The model under review builds one solid part; all positions refer to its coordinate system, in mm. Face numbers are marked on the shaded views. A direction names the side the tool comes from. Give positions to 0.01 mm unless a question says otherwise; leave off trailing zeros. Order: outer loops, then holes, each group sorted by start corner. A loop starts at its lowest first (then second) coordinate and runs counter-clockwise, first axis right, second up. Notation, with made-up numbers: (-23.75, 83) - (6.25, 83) arc R12 ccw to (6.25, 99) - close; hole circle Ø4 at (46, 24). An arc over 180 degrees is marked (long way). Answer as CSV lines item,"result". Start each with the question number.
from build123d import *

# Parameters (mm, degrees)
SKETCH1_R           = 9.5
BOSS_EXTRUDE1_DEPTH = 68
SKETCH2_R           = 8
BOSS_EXTRUDE2_DEPTH = 28
SKETCH3_R           = 7
BOSS_EXTRUDE3_DEPTH = 22
SKETCH4_R           = 6
BOSS_EXTRUDE4_DEPTH = 10
SKETCH5_R           = 37.5
BOSS_EXTRUDE5_DEPTH = 1.5
SKETCH6_R           = 12.5
SKETCH6_R_2         = 7
BOSS_EXTRUDE6_DEPTH = 17.5
FILLET1_R           = 6
BOSS_EXTRUDE7_DEPTH = 14
FILLET2_R           = 3


with BuildPart() as part:
    # Sketch1 → Boss-Extrude1 (new body)
    with BuildSketch(Plane.XY):
        Circle(SKETCH1_R)
    extrude(amount=BOSS_EXTRUDE1_DEPTH)

    # Sketch2 → Boss-Extrude2 (add)
    with BuildSketch(Plane.XY.offset(68)):
        Circle(SKETCH2_R)
    extrude(amount=BOSS_EXTRUDE2_DEPTH)

    # Sketch3 → Boss-Extrude3 (add)
    with BuildSketch(Plane.XY.offset(96)):
        Circle(SKETCH3_R)
    extrude(amount=BOSS_EXTRUDE3_DEPTH)

    # Sketch4 → Boss-Extrude4 (add)
    with BuildSketch(Plane.XY.offset(118)):
        Circle(SKETCH4_R)
    extrude(amount=BOSS_EXTRUDE4_DEPTH)

    # Sketch5 → Boss-Extrude5 (add)
    with BuildSketch(Plane(origin=(0, 0, 0), x_dir=(-1, 0, 0), z_dir=(0, 0, -1))):
        Circle(SKETCH5_R)
    extrude(amount=BOSS_EXTRUDE5_DEPTH)

    # Sketch6 → Boss-Extrude6 (add)
    with BuildSketch(Plane(origin=(0, 0, -1.5), x_dir=(-1, 0, 0), z_dir=(0, 0, -1))):
        Circle(SKETCH6_R)
        Circle(SKETCH6_R_2, mode=Mode.SUBTRACT)
    extrude(amount=BOSS_EXTRUDE6_DEPTH)

    # Fillet1
    fillet1_edges = [part.edges().sort_by_distance(p)[0] for p in [
        (12.5, 0, -1.5),
    ]]
    fillet(fillet1_edges, radius=FILLET1_R)

    # Sketch8 → Boss-Extrude7 (add)
    with BuildSketch(Plane.XY):
        with BuildLine():
            ThreePointArc((-14.519262929, -12.255243939), (-13.410586975, -13.459426325), (-12.202382266, -14.563717487))
            ThreePointArc((-12.202382266, -14.563717487), (-23.134563913, -16.979972169), (-34.212072677, -15.355262394))
            ThreePointArc((-34.212072677, -15.355262394), (-34.993730727, -13.479199154), (-35.672601083, -11.563543228))
            ThreePointArc((-35.672601083, -11.563543228), (-25.163804407, -13.985042516), (-14.519262929, -12.255243939))
        make_face()
        with BuildLine():
            ThreePointArc((7.821978348, 36.675150371), (0.470500112, 28.78501513), (-3.353721116, 18.70167251))
            ThreePointArc((-3.353721116, 18.70167251), (-4.95091163, 18.343622162), (-6.511358184, 17.849431772))
            ThreePointArc((-6.511358184, 17.849431772), (-3.137805297, 28.525106139), (3.807989024, 37.306155251))
            ThreePointArc((3.807989024, 37.306155251), (5.823536473, 37.045059359), (7.821978348, 36.675150371))
        make_face()
        with BuildLine():
            ThreePointArc((-27.850622735, 25.111607143), (-24.693304295, 14.799972614), (-17.872984045, 6.446428571))
            ThreePointArc((-17.872984045, 6.446428571), (-18.361498605, 4.884195838), (-18.71374045, 3.285714286))
            ThreePointArc((-18.71374045, 3.285714286), (-26.27236921, 11.54513397), (-30.404083653, 21.950892857))
            ThreePointArc((-30.404083653, 21.950892857), (-29.170194253, 23.565860206), (-27.850622735, 25.111607143))
        make_face()
        with BuildLine():
            ThreePointArc((35.672601083, 11.563543228), (25.163804407, 13.985042516), (14.519262929, 12.255243939))
            ThreePointArc((14.519262929, 12.255243939), (13.410586975, 13.459426325), (12.202382266, 14.563717487))
            ThreePointArc((12.202382266, 14.563717487), (23.134563913, 16.979972169), (34.212072677, 15.355262394))
            ThreePointArc((34.212072677, 15.355262394), (34.993730727, 13.479199154), (35.672601083, 11.563543228))
        make_face()
        with BuildLine():
            ThreePointArc((27.850622735, -25.111607143), (24.693304295, -14.799972614), (17.872984045, -6.446428571))
            ThreePointArc((17.872984045, -6.446428571), (18.361498605, -4.884195838), (18.71374045, -3.285714286))
            ThreePointArc((18.71374045, -3.285714286), (26.27236921, -11.54513397), (30.404083653, -21.950892857))
            ThreePointArc((30.404083653, -21.950892857), (29.170194253, -23.565860206), (27.850622735, -25.111607143))
        make_face()
        with BuildLine():
            ThreePointArc((-7.821978348, -36.675150371), (-0.470500112, -28.78501513), (3.353721116, -18.70167251))
            ThreePointArc((3.353721116, -18.70167251), (4.95091163, -18.343622162), (6.511358184, -17.849431772))
            ThreePointArc((6.511358184, -17.849431772), (3.137805297, -28.525106139), (-3.807989024, -37.306155251))
            ThreePointArc((-3.807989024, -37.306155251), (-5.823536473, -37.045059359), (-7.821978348, -36.675150371))
        make_face()
    extrude(amount=BOSS_EXTRUDE7_DEPTH)

    # Fillet2
    fillet2_edges = [part.edges().sort_by_distance(p)[0] for p in [
        (-18.361498605, 4.884195838, 0),
        (-4.95091163, 18.343622162, 0),
        (13.410586975, 13.459426325, 0),
        (18.361498605, -4.884195838, 0),
        (4.95091163, -18.343622162, 0),
        (-13.410586975, -13.459426325, 0),
    ]]
    fillet(fillet2_edges, radius=FILLET2_R)


solid = part.part
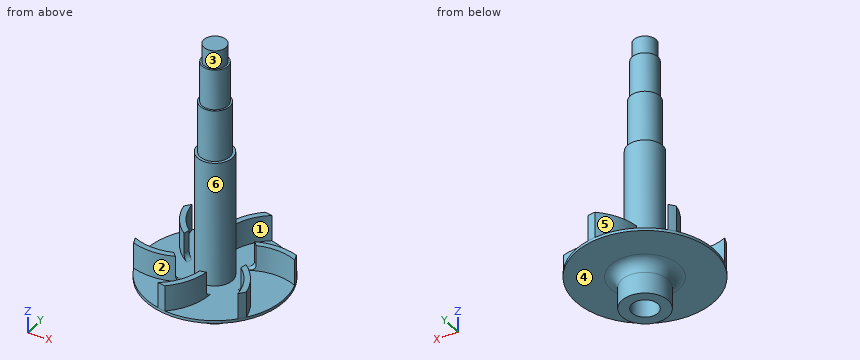
Item 1: Machinability: for the marked faces 4, 5 and 6, which of the approach directions +Z, -Z, +X, -X, +Y, -Y give a long, thin tool a straight path to every point of the face, cutting with its end or side? Answer none if there is none.
Item 2: Mouldability with a two-part tool opening along Y and no side actions: class the marked faces 1, 2 and 3 as released by +Y, released by -Y, zero draft, split by the parting line, or undercut.
Item 3: For line 1 along Y through (x, z) = (0, -10); line 2 along Z through (x, y) = (-24, -12.5); line 3 along Y through (x, z) = (5.5, -6), list the stretches that pass through material, from the lowest coordinate up.
Item 4: Clearance check with flat-ended pins moving along their axes: pin 1 (7 mm diameter, centred on x = 1, y = 25.5, fed in from +Z); pin 2 (4 mm diameter, centred on x = 1.5, y = 1.5, fed in from -Z); pin 3 (4 mm diameter, centred on x = -10.5, y = 19, fed in from +Z). State where each tip first meets the part, or that it passes through.
Item 5: Take a section at B-B on y = 29.5. Write out the cut boundary in (x, z), and give its area (3 significant figures).
Item 6: Take a section at A-A on z = 64. Write out the cut boundary in (x, y).
Data:
1,face 4,"-Z"
1,face 5,"+Z, +Y"
1,face 6,"+Z"
2,face 1,"undercut"
2,face 2,"released by -Y"
2,face 3,"split by the parting line"
3,line 1,"y = -12.5 to -7, 7 to 12.5"
3,line 2,"z = -1.5 to 0"
3,line 3,"y = -11.44 to -4.33, 4.33 to 11.44"
4,pin 1,"stops at z = 14"
4,pin 2,"stops at z = -1.5"
4,pin 3,"stops at z = 0"
5,outline,"(-23.15, -1.5) - (23.15, -1.5) - (23.15, 0) - (0.93, 0) - (0.93, 14) - (-2.6, 14) - (-2.6, 0) - (-23.15, 0) - close"
5,area,"119 mm^2"
6,outline,"circle Ø19 at (0, 0)"
